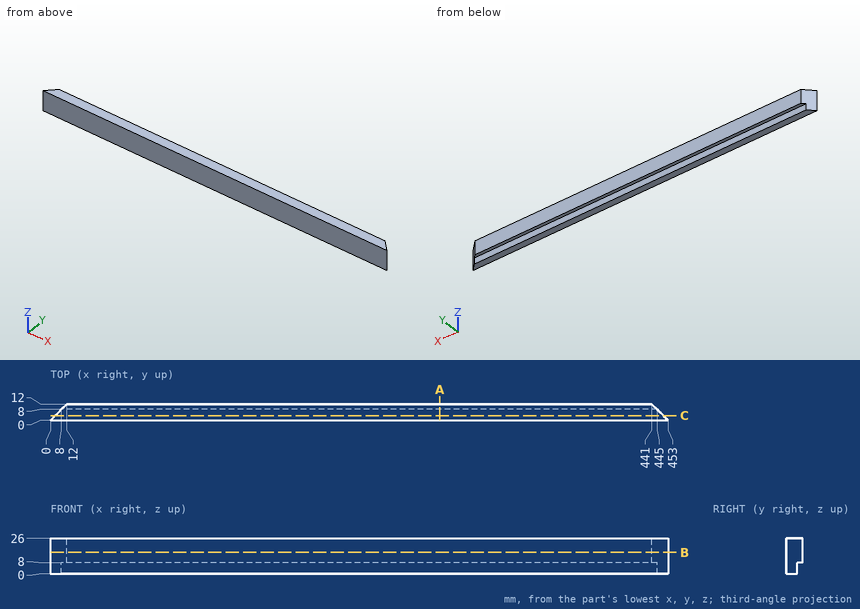
Geometry check sheet. Reference: drawing and pictorial views, mm from the part's lowest x, y, z. Coordinates: 2 decimals unless noted, no trailing zeros. Order: outer loops, then holes, each group sorted by start corner. A loop starts at its lowest first (then second) coordinate and runs counter-clockwise, first axis right, second up.
Item 1: Section check A-A, the plane x = 285.5. Enter the section's corners in (y, z), then the cut area to 3 significant figures.
Filled in:
outline: (0, 0) - (8, 0) - (8, 8) - (12, 8) - (12, 26) - (0, 26) - close
area: 280 mm2
Item 2: Section check B-B, the plane z = 15.75. Enter the section's corners in (x, y), then the cut area to 3 significant figures.
Filled in:
outline: (0, 0) - (453, 0) - (441, 12) - (12, 12) - close
area: 5,290 mm2
Item 3: Material ranges on L1, parallel to Z at x = 203, y = 8.5; L2, parallel to Y at x = 250, z = 1.5; L3, parallel to X at y = 9.5, z = 18.75, recorded low to high.
Filled in:
L1: z = 8 to 26
L2: y = 0 to 8
L3: x = 9.5 to 443.5
Item 4: Depth check by flat-ended pin: pin 1 (3 mm diameter, centred on x = 321, y = 11, fed in from -Z); pin 2 (4 mm diameter, centred on y = 3, z = 21.5, fed in from +X). Enter the tip coordinate at first touch or a pass-through.
Filled in:
pin 1: stops at z = 8
pin 2: stops at x = 452
Item 5: Section check C-C, the plane y = 3.5. Enter the section's corners in (x, z), then the cut area to 3 significant figures.
Filled in:
outline: (3.5, 0) - (449.5, 0) - (449.5, 26) - (3.5, 26) - close
area: 11,600 mm2
